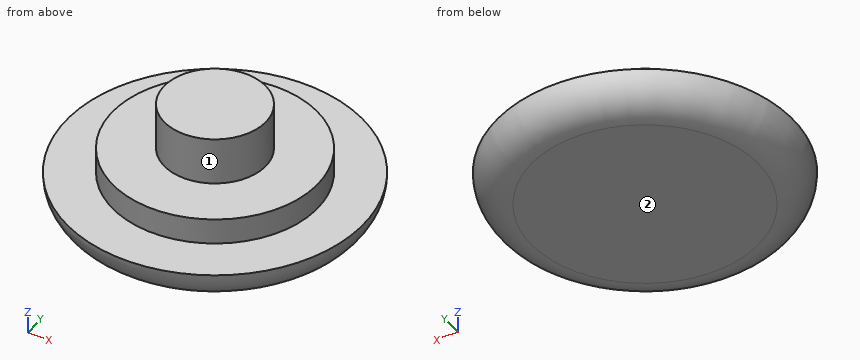
from build123d import *

# Parameters (mm, degrees)
F0_R     = 8.6
F0_R_2   = 5.95
F1_DEPTH = 2
F0_R_3   = 2.95
F2_DEPTH = 3.5
F3_DEPTH = 6.25
F4_R     = 1.99999


# Not quite as in the source:
# - a fillet or chamfer is up to 0.001 mm smaller than in the source, because OpenCascade refuses the exact size
# - a feature names something its author has since deleted; it is built from what else it names


with BuildPart() as f1:
    # F0 (on Top) → F1 (new body)
    with BuildSketch(Plane.XY):
        with Locations((-45.6172116101, 18.5634717345)):
            Circle(F0_R)
        with Locations((-45.6172116101, 18.5634717345)):
            Circle(F0_R_2, mode=Mode.SUBTRACT)
    extrude(amount=F1_DEPTH)

    # F0 (on Top) → F2 (join)
    with BuildSketch(Plane.XY):
        with Locations((-45.6172116101, 18.5634717345)):
            Circle(F0_R_2)
        with Locations((-45.6172116101, 18.5634717345)):
            Circle(F0_R_3, mode=Mode.SUBTRACT)
    extrude(amount=F2_DEPTH)

    # F0 (on Top) → F3 (join)
    with BuildSketch(Plane.XY):
        with Locations((-45.6172116101, 18.5634717345)):
            Circle(F0_R_3)
    extrude(amount=F3_DEPTH)

    # F4 (radius 2 in the source; OpenCascade refuses exactly that, so slightly less here)
    f4_edges = [f1.edges().sort_by_distance(p)[0] for p in [
        (-54.217212, 18.563472, 0),
    ]]
    fillet(f4_edges, radius=F4_R)


solid = f1.part
Geometry: final body of the model. Coordinates: model frame, mm. Face numbers are marked on the shaded views. A direction names the side the tool comes from. Give positions to 0.01 mm unless a question says otherwise; leave off trailing zeros. Write each loop counter-clockwise with the first axis right and the second up, starting at its lowest first coordinate (ties: lowest second). Pieces come first, ordered by that corner, then holes. Notation, with made-up numbers: (-20, 12.25) -> (-1, 12.25) arc R23 ccw to (-1, 51.25) -> close; hole circle Ø11 at (71.5, 53.25). An arc over 180 degrees is marked (long way). Answer as a JSON object with one key per item and string values.
1. Cut plane B-B on z = 4.5. Output: boundary loops of the cut face in (x, y).
Ans:
{"outline": "circle Ø5.9 at (-45.62, 18.56)"}
2. Ray query, probe 1 along Z at (x, y) = (-48.75, 23.5); probe 2 along Z at (x, y) = (-51.75, 18.5); probe 3 along Y at (x, z) = (-50.25, 3). Return the intervals inside material, ascending. Write a range as from..to.
Ans:
{"probe 1": "z = 0..3.5", "probe 2": "z = 0..2", "probe 3": "y = 14.83..22.3"}
3. Access query for the marked faces 1 and 2. Directions: +Z, -Z, +X, -X, +Y, -Y. A direction counts if a zero-diameter tool reaches every point of the face in a straight line with its end or side. Return the directions, or none.
Ans:
{"face 1": "+Z", "face 2": "-Z, +X, -X, +Y, -Y"}
4. Cut plane A-A on z = 1.5. Output: boundary loops of the cut face in (x, y).
Ans:
{"outline": "circle Ø17.07 at (-45.62, 18.56)"}
5. Contact query for a flat-ended pin moving along its axis: pin 1 (1 mm diameter, centred on x = -41, z = 2, fed in from +Y). Output: stop coordinate, or through.
Ans:
{"pin 1": "stops at y = 26.11"}
